Input: dimensioned drawing with shaded views. Units: mm. Origin: part minimum x, y, z. Coordinates: 2 decimals unless noted, no trailing zeros. Loops run counter-clockwise (first coordinate to the right, second up) from the corner with the lowest first, then second, coordinate; pieces in that order, holes last.
Item 1: Section A-A on y = 5.75. Return loops of the section in (x, z), and give its area (3 significant figures).
Item 2: Section C-C on z = 7.5. Return loops of the section in (x, y).
Item 3: Section B-B on x = 11. Return loops of the section in (y, z), and give its area (3 significant figures).
Item 4: Ray query, line 1 along Z through (x, y) = (11, 2.5); line 2 along X through (y, z) = (3, 42.5); line 3 along Y through (x, z) = (1.75, 13.5). Return the intervals inside material, ascending.
Item 5: Section D-D on x = 18.25. Return loops of the section in (y, z).
Item 6: Contact query for flat-ended pins moving along their axis: P1, Ø2, axis at y = 4.5, z = 12, coming from the +X side; P2, Ø3, axis at x = 6, z = 33, coming from the -Y side; P3, Ø1, axis at y = 5, z = 18.5, coming from the -X side. Output: stop coordinate, or through.
Item 7: Pull-direction query (X, two-part tool) for the marked faces 1, 2 and 3; classes: released by +X, released by -X, zero draft, split by the parting line, or undercut.
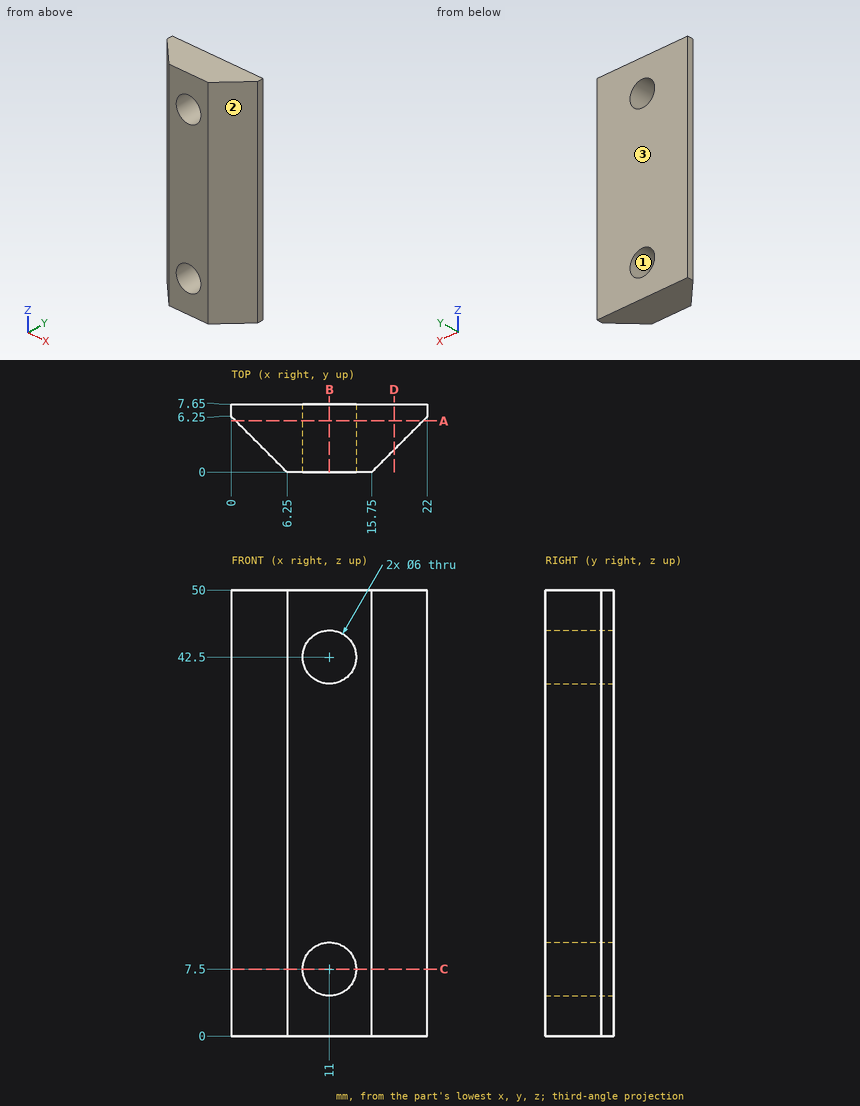
Results found:
1. outline: (0.5, 0) - (21.5, 0) - (21.5, 50) - (0.5, 50) - close; hole circle Ø6 at (11, 7.5); hole circle Ø6 at (11, 42.5)
1. area: 993 mm2
2. outline: (0, 6.25) - (6.25, 0) - (8, 0) - (8, 7.65) - (0, 7.65) - close; (14, 0) - (15.75, 0) - (22, 6.25) - (22, 7.65) - (14, 7.65) - close
3. outline: (0, 0) - (7.65, 0) - (7.65, 4.5) - (0, 4.5) - close; (0, 10.5) - (7.65, 10.5) - (7.65, 39.5) - (0, 39.5) - close; (0, 45.5) - (7.65, 45.5) - (7.65, 50) - (0, 50) - close
3. area: 291 mm2
4. line 1: z = 0 to 4.5, 10.5 to 39.5, 45.5 to 50
4. line 2: x = 3.25 to 8, 14 to 18.75
4. line 3: y = 4.5 to 7.65
5. outline: (2.5, 0) - (7.65, 0) - (7.65, 50) - (2.5, 50) - close
6. P1: stops at x = 21.25
6. P2: stops at y = 0
6. P3: stops at x = 0.75
7. face 1: undercut
7. face 2: released by +X
7. face 3: zero draft
